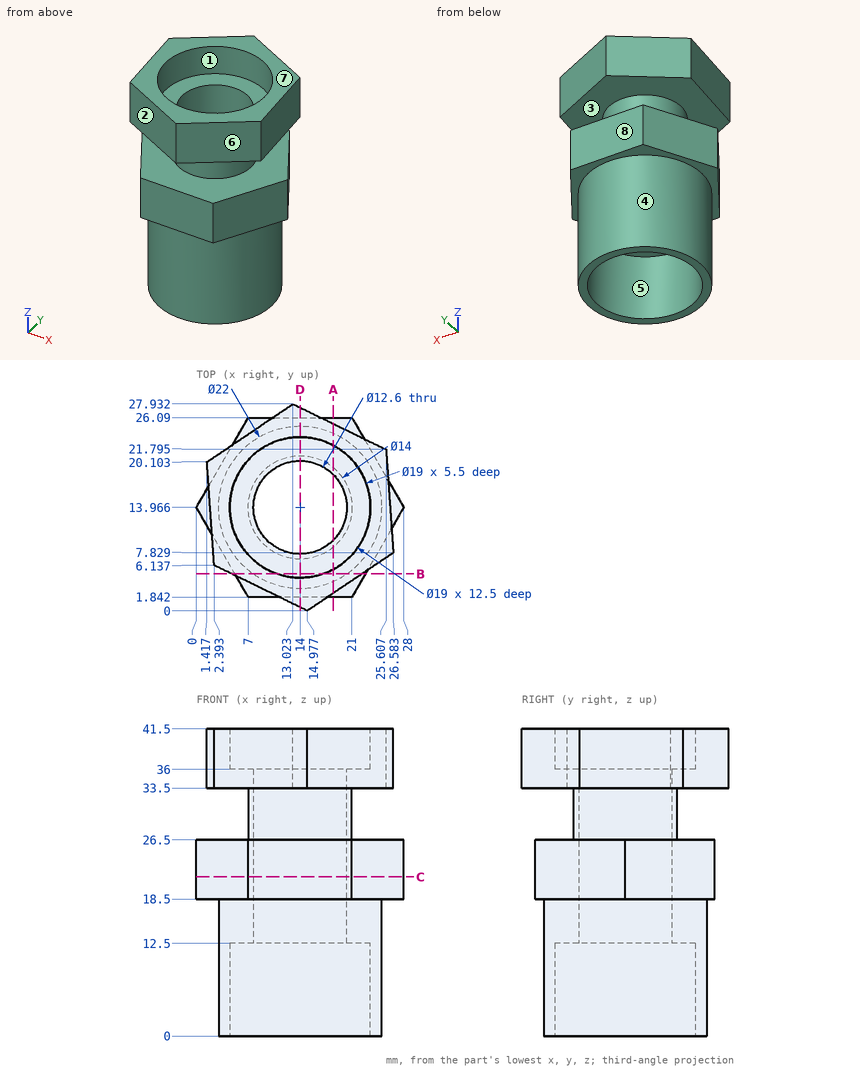
Study the drawing (mm; zero at the part's minimum x, y, z) and answer. A direction names the side the tool comes from. Coordinates: 2 decimals unless noted, no trailing zeros. Loops run counter-clockwise (first coordinate to the right, second up) from the corner with the lowest first, then second, coordinate; pieces in that order, holes last. Notation, with made-up numbers: M 84.25,65.5 L 130.25,65.5 A19 cw 130.25,91.5 Z; hole C -38,-14.75 d1. An arc over 180 degrees is marked long. Answer as a JSON object with one key per item and string values. Group by question number.
Item 1: Consider L1, parallel to Z at x = 12, y = 5.25; L2, parallel to Y at x = 14, z = 26.75 (1 decimal); L3, parallel to Z at x = 5.5, y = 5.75. Determine where each line is inside the solid, lowest interval first.
Item 2: Section B-B (y = 5) is taken. Write down the section's boundary in (x, z) (1 decimal), and give its area (3 significant figures).
Item 3: Section C-C (z = 21.5) is taken. Write down the section's boundary in (x, y) (1 decimal).
Item 4: Each of these flat-tipped pins is pushed along its axis until it touches: P1, Ø9, axis at x = 11.5, z = 20.5, coming from the -Y side; P2, Ø5, axis at x = 15, z = 6, coming from the -Y side; P3, Ø6.5, axis at x = 13.5, z = 24.5, coming from the +Y side. Where does it stop, or does it pass through?
Item 5: Section A-A (x = 18.5) is taken. Write down the section's boundary in (y, z) (1 decimal), and give its area (3 significant figures).
Item 6: Section D-D (x = 14) is taken. Write down the section's boundary in (y, z) (1 decimal).
Item 7: Determine the mould class of the marked faces 5, 6, 7 and 8 for opening direction Y: +Y half, -Y half, draft (parallel to the pull), parting line (faces both ways), or undercut.
Item 8: Which of the six approach directions +Z, -Z, +X, -X, +Y, -Y give full straight-line access (tool end or side, diameter ignored) to the marked faces 1, 2, 3 and 4?
Solved:
{
 "1": {"L1": "z = 12.5 to 26.5, 33.5 to 36", "L2": "y = 7 to 7.7, 20.3 to 21", "L3": "z = 18.5 to 26.5, 33.5 to 41.5"},
 "2": {"outline": "M 4.7,33.5 L 22.4,33.5 L 22.4,41.5 L 17.1,41.5 L 17.1,36 L 10.9,36 L 10.9,41.5 L 4.7,41.5 Z; M 5.2,18.5 L 7.6,18.5 L 7.6,0 L 10.9,0 L 10.9,12.5 L 17.1,12.5 L 17.1,0 L 20.4,0 L 20.4,18.5 L 22.8,18.5 L 22.8,26.5 L 5.2,26.5 Z", "area": "405 mm2"},
 "3": {"outline": "M 0,14 L 7,1.8 L 21,1.8 L 28,14 L 21,26.1 L 7,26.1 Z; hole C 14,14 d12.6"},
 "4": {"P1": "stops at y = 1.84", "P2": "stops at y = 2.97", "P3": "stops at y = 26.09"},
 "5": {"outline": "M 1.8,18.5 L 3.9,18.5 L 3.9,0 L 5.6,0 L 5.6,12.5 L 9.6,12.5 L 9.6,36 L 5.6,36 L 5.6,41.5 L 2.4,41.5 L 2.4,33.5 L 8.6,33.5 L 8.6,26.5 L 1.8,26.5 Z; M 18.4,12.5 L 22.3,12.5 L 22.3,0 L 24,0 L 24,18.5 L 26.1,18.5 L 26.1,26.5 L 19.3,26.5 L 19.3,33.5 L 25.3,33.5 L 25.3,41.5 L 22.3,41.5 L 22.3,36 L 18.4,36 Z", "area": "315 mm2"},
 "6": {"outline": "M 0.5,33.5 L 7,33.5 L 7,26.5 L 1.8,26.5 L 1.8,18.5 L 3,18.5 L 3,0 L 4.5,0 L 4.5,12.5 L 7.7,12.5 L 7.7,36 L 4.5,36 L 4.5,41.5 L 0.5,41.5 Z; M 20.3,12.5 L 23.5,12.5 L 23.5,0 L 25,0 L 25,18.5 L 26.1,18.5 L 26.1,26.5 L 21,26.5 L 21,33.5 L 27.5,33.5 L 27.5,41.5 L 23.5,41.5 L 23.5,36 L 20.3,36 Z"},
 "7": {"face 5": "undercut", "face 6": "-Y half", "face 7": "draft", "face 8": "+Y half"},
 "8": {"face 1": "+Z", "face 2": "+Z, -X, -Y", "face 3": "none", "face 4": "-Z"}
}
